The model under review builds one solid part; all positions refer to its coordinate system, in mm. Round coordinates to 2 decimals unless told otherwise and drop trailing zeros. Write each loop counter-clockwise with the first axis right and the second up, starting at its lowest first coordinate (ties: lowest second). Pieces come first, ordered by that corner, then holes. Notation, with made-up numbers: M 66,37.25 L 110,37.25 A18 ccw 110,64.25 Z; hole C 40,-21 d8. An arc over 180 degrees is marked long. One line per item, written item: value. Start each with the question number.
1) Take a section at B-B, the plane z = 72.5. Write out the cut boundary in (x, y).
2) For P1, Ø3.5, axis at x = -47.5, z = 32, coming from the -Y side; P2, Ø3, axis at x = 15, z = 12.5, coming from the -Y side; P3, Ø1.5, axis at x = 58.5, y = 1.5, coming from the +Z side, all flat-tipped, find the tip position at first contact; note any pin that passes through.
3) Wall thickness on probe 1 along Z at (x, y) = (62, 2.65); probe 2 along X at (y, z) = (2.6, -17); probe 3 along X at (y, z) = (0.6, -47.5): over which ranges is each line inside the solid? List them lowest first.
4) Take a section at D-D, the plane z = 14. Write out the cut boundary in (x, y).
5) Take a section at A-A, the plane x = 47.5. Write out the cut boundary in (y, z).
6) Take a section at C-C, the plane x = 62. Write out the cut boundary in (y, z), and give its area (3 significant figures).
from build123d import *

# Parameters (mm, degrees)
SKETCH1_W               = 139
SKETCH1_H               = 160
BOSS_EXTRUDE1_DEPTH     = 5
SKETCH2_W               = 16
SKETCH2_H               = 16
CUT_EXTRUDE1_DEPTH      = 107.090763029
SKETCH3_R               = 2.2
CUT_EXTRUDE2_DEPTH      = 107.090763029
SKETCH4_R               = 2.2
CUT_EXTRUDE3_DEPTH      = 107.090763029
LPATTERN1_COUNT         = 4
LPATTERN1_PITCH         = 35
MIRROR2_COPY_1_SKETCH_R = 2.2
MIRROR2_COPY_1_DEPTH    = 107.090763029
MIRROR2_COPY_2_SKETCH_R = 2.2
MIRROR2_COPY_2_DEPTH    = 107.090763029
MIRROR2_COPY_3_SKETCH_R = 2.2
MIRROR2_COPY_3_DEPTH    = 107.090763029
SKETCH5_R               = 2.2
CUT_EXTRUDE4_DEPTH      = 107.090763029
CUT_EXTRUDE5_DEPTH      = 107.090763029


with BuildPart() as part:
    # Sketch1 → Boss-Extrude1 (new body)
    with BuildSketch(Plane(origin=(0, 0, 0), x_dir=(1, 0, 0), z_dir=(0, 1, 0))):
        Rectangle(SKETCH1_W, SKETCH1_H)
    extrude(amount=BOSS_EXTRUDE1_DEPTH)

    # Sketch2 → Cut-Extrude1 (cut, through all)
    with BuildSketch(Plane(origin=(0, 5, 0), x_dir=(1, 0, 0), z_dir=(0, 1, 0))):
        with Locations((-61.5, -72)):
            Rectangle(SKETCH2_W, SKETCH2_H)
    cut_extrude1 = extrude(amount=-CUT_EXTRUDE1_DEPTH, mode=Mode.SUBTRACT)

    # Mirror1: Cut-Extrude1 across plane
    add(cut_extrude1.mirror(Plane(origin=(0, 0, 0), x_dir=(0, 0, 1), z_dir=(1, 0, 0))), mode=Mode.SUBTRACT)

    # Sketch3 → Cut-Extrude2 (cut, through all)
    with BuildSketch(Plane(origin=(0, 5, 0), x_dir=(1, 0, 0), z_dir=(0, 1, 0))):
        with Locations(Location((0, -72.5, 0), (0, 0, 270))):
            Circle(SKETCH3_R)
        with Locations(Location((-25, -72.5, 0), (0, 0, 270))):
            Circle(SKETCH3_R)
        with Locations(Location((25, -72.5, 0), (0, 0, 270))):
            Circle(SKETCH3_R)
    extrude(amount=-CUT_EXTRUDE2_DEPTH, mode=Mode.SUBTRACT)

    # Sketch4 → Cut-Extrude3 (cut, through all)
    with BuildSketch(Plane(origin=(0, 5, 0), x_dir=(1, 0, 0), z_dir=(0, 1, 0))):
        with Locations(Location((-62, -49, 0), (0, 0, 270))):
            Circle(SKETCH4_R)
    cut_extrude3 = extrude(amount=-CUT_EXTRUDE3_DEPTH, mode=Mode.SUBTRACT)

    # LPattern1: Cut-Extrude3 ×4
    with Locations(*[(0, 0, -i * LPATTERN1_PITCH) for i in range(1, LPATTERN1_COUNT)]):
        add(cut_extrude3, mode=Mode.SUBTRACT)

    # Mirror2: Cut-Extrude3 across plane
    add(cut_extrude3.mirror(Plane(origin=(0, 0, 0), x_dir=(0, 0, 1), z_dir=(1, 0, 0))), mode=Mode.SUBTRACT)

    # Mirror2 copy 1 sketch → Mirror2 copy 1 (cut, through all)
    with BuildSketch(Plane(origin=(0, 5, -35), x_dir=(-1, 0, 0), z_dir=(0, 1, 0))):
        with Locations((-62, 49)):
            Circle(MIRROR2_COPY_1_SKETCH_R)
    extrude(amount=-MIRROR2_COPY_1_DEPTH, mode=Mode.SUBTRACT)

    # Mirror2 copy 2 sketch → Mirror2 copy 2 (cut, through all)
    with BuildSketch(Plane(origin=(0, 5, -70), x_dir=(-1, 0, 0), z_dir=(0, 1, 0))):
        with Locations((-62, 49)):
            Circle(MIRROR2_COPY_2_SKETCH_R)
    extrude(amount=-MIRROR2_COPY_2_DEPTH, mode=Mode.SUBTRACT)

    # Mirror2 copy 3 sketch → Mirror2 copy 3 (cut, through all)
    with BuildSketch(Plane(origin=(0, 5, -105), x_dir=(-1, 0, 0), z_dir=(0, 1, 0))):
        with Locations((-62, 49)):
            Circle(MIRROR2_COPY_3_SKETCH_R)
    extrude(amount=-MIRROR2_COPY_3_DEPTH, mode=Mode.SUBTRACT)

    # Sketch5 → Cut-Extrude4 (cut, through all)
    with BuildSketch(Plane(origin=(0, 5, 0), x_dir=(1, 0, 0), z_dir=(0, 1, 0))):
        with Locations(Location((-47.5, -32, 0), (0, 0, 270))):
            Circle(SKETCH5_R)
        with Locations(Location((-47.5, -7, 0), (0, 0, 270))):
            Circle(SKETCH5_R)
    cut_extrude4 = extrude(amount=-CUT_EXTRUDE4_DEPTH, mode=Mode.SUBTRACT)

    # Mirror3: Cut-Extrude4 across plane
    add(cut_extrude4.mirror(Plane(origin=(0, 0, 0), x_dir=(0, 0, 1), z_dir=(1, 0, 0))), mode=Mode.SUBTRACT)

    # Sketch6 → Cut-Extrude5 (cut, through all)
    with BuildSketch(Plane(origin=(0, 5, 0), x_dir=(1, 0, 0), z_dir=(0, 1, 0))):
        Polygon((0, 50), (-10, 32.679491924), (10, 32.679491924), align=None)
        Polygon((15, 50), (25, 32.679491924), (35, 50), align=None)
        Polygon((-25, 32.679491924), (-35, 50), (-15, 50), align=None)
        Polygon((25, 22.679491924), (35, 5.358983849), (15, 5.358983849), align=None)
        Polygon((-10, 22.679491924), (10, 22.679491924), (0, 5.358983849), align=None)
        Polygon((-15, 5.358983849), (-25, 22.679491924), (-35, 5.358983849), align=None)
        Polygon((15, -5.358983849), (25, -22.679491924), (35, -5.358983849), align=None)
        Polygon((0, -5.358983849), (-10, -22.679491924), (10, -22.679491924), align=None)
        Polygon((-35, -5.358983849), (-15, -5.358983849), (-25, -22.679491924), align=None)
        Polygon((25, -32.679491924), (35, -50), (15, -50), align=None)
        Polygon((-10, -32.679491924), (10, -32.679491924), (0, -50), align=None)
        Polygon((-15, -50), (-25, -32.679491924), (-35, -50), align=None)
    extrude(amount=-CUT_EXTRUDE5_DEPTH, mode=Mode.SUBTRACT)


solid = part.part
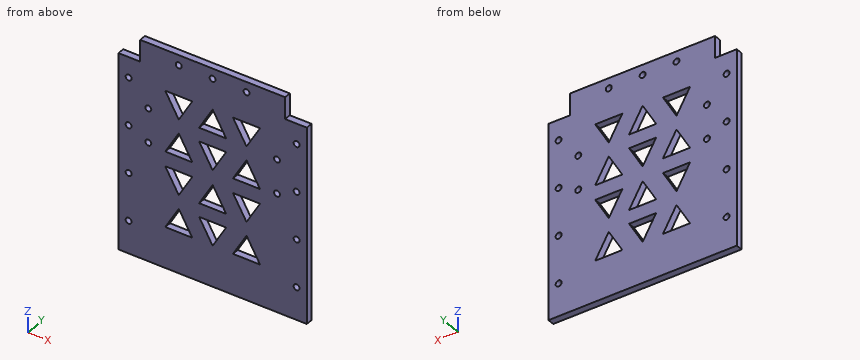
Checked values:
1. outline: M -53.5,0 L -27.2,0 L -27.2,5 L -53.5,5 Z; M -22.8,0 L -2.2,0 L -2.2,5 L -22.8,5 Z; M 2.2,0 L 22.8,0 L 22.8,5 L 2.2,5 Z; M 27.2,0 L 53.5,0 L 53.5,5 L 27.2,5 Z
2. P1: passes through
2. P2: stops at y = 0
2. P3: stops at z = 64
3. probe 1: z = -80 to -58.2, -53.8 to -23.2, -18.8 to 11.8, 16.2 to 46.8, 51.2 to 64
3. probe 2: x = -69.5 to -28.28, -21.72 to -6.72, 6.72 to 21.72, 28.28 to 69.5
3. probe 3: x = -69.5 to -33.56, -16.44 to -1.44, 1.44 to 16.44, 33.56 to 69.5
4. outline: M -69.5,0 L -64.2,0 L -64.2,5 L -69.5,5 Z; M -59.8,0 L -30.01,0 L -30.01,5 L -59.8,5 Z; M -19.99,0 L -4.99,0 L -4.99,5 L -19.99,5 Z; M 4.99,0 L 19.99,0 L 19.99,5 L 4.99,5 Z; M 30.01,0 L 59.8,0 L 59.8,5 L 30.01,5 Z; M 64.2,0 L 69.5,0 L 69.5,5 L 64.2,5 Z
5. outline: M 0,-80 L 5,-80 L 5,4.8 L 0,4.8 Z; M 0,9.2 L 5,9.2 L 5,29.8 L 0,29.8 Z; M 0,34.2 L 5,34.2 L 5,80 L 0,80 Z
6. outline: M 0,-80 L 5,-80 L 5,-58.2 L 0,-58.2 Z; M 0,-53.8 L 5,-53.8 L 5,-23.2 L 0,-23.2 Z; M 0,-18.8 L 5,-18.8 L 5,11.8 L 0,11.8 Z; M 0,16.2 L 5,16.2 L 5,46.8 L 0,46.8 Z; M 0,51.2 L 5,51.2 L 5,64 L 0,64 Z
6. area: 632 mm2
